```python
from build123d import *

# Parameters (mm, degrees)
F1_DEPTH = 20
F2_DEPTH = 5
F3_W     = 60
F3_H     = 100
F4_DEPTH = 0.5


with BuildPart() as f1:
    # F0 (on Top) → F1 (new body)
    with BuildSketch(Plane.XY):
        with BuildLine():
            Line((45, -47.5), (45, 47.5))
            ThreePointArc((45, 47.5), (39.874369, 59.874369), (27.5, 65))
            Line((27.5, 65), (-27.5, 65))
            ThreePointArc((-27.5, 65), (-39.874369, 59.874369), (-45, 47.5))
            Line((-45, 47.5), (-45, -47.5))
            ThreePointArc((-45, -47.5), (-39.874369, -59.874369), (-27.5, -65))
            Line((-27.5, -65), (27.5, -65))
            ThreePointArc((27.5, -65), (39.874369, -59.874369), (45, -47.5))
        make_face()
        with BuildLine():
            Line((-27.5, 62.5), (27.5, 62.5))
            ThreePointArc((27.5, 62.5), (38.106602, 58.106602), (42.5, 47.5))
            Line((42.5, 47.5), (42.5, -47.5))
            ThreePointArc((42.5, -47.5), (38.106602, -58.106602), (27.5, -62.5))
            Line((27.5, -62.5), (-27.5, -62.5))
            ThreePointArc((-27.5, -62.5), (-38.106602, -58.106602), (-42.5, -47.5))
            Line((-42.5, -47.5), (-42.5, 47.5))
            ThreePointArc((-42.5, 47.5), (-38.106602, 58.106602), (-27.5, 62.5))
        make_face(mode=Mode.SUBTRACT)
    extrude(amount=F1_DEPTH)

    # F0 (on Top) → F2 (join)
    with BuildSketch(Plane.XY):
        with BuildLine():
            ThreePointArc((42.5, 47.5), (38.106602, 58.106602), (27.5, 62.5))
            Line((27.5, 62.5), (-27.5, 62.5))
            ThreePointArc((-27.5, 62.5), (-38.106602, 58.106602), (-42.5, 47.5))
            Line((-42.5, 47.5), (-42.5, -47.5))
            ThreePointArc((-42.5, -47.5), (-38.106602, -58.106602), (-27.5, -62.5))
            Line((-27.5, -62.5), (27.5, -62.5))
            ThreePointArc((27.5, -62.5), (38.106602, -58.106602), (42.5, -47.5))
            Line((42.5, -47.5), (42.5, 47.5))
        make_face()
        with BuildLine():
            Line((-20, 47.5), (20, 47.5))
            ThreePointArc((20, 47.5), (25.303301, 45.303301), (27.5, 40))
            Line((27.5, 40), (27.5, -40))
            ThreePointArc((27.5, -40), (25.303301, -45.303301), (20, -47.5))
            Line((20, -47.5), (-20, -47.5))
            ThreePointArc((-20, -47.5), (-25.303301, -45.303301), (-27.5, -40))
            Line((-27.5, -40), (-27.5, 40))
            ThreePointArc((-27.5, 40), (-25.303301, 45.303301), (-20, 47.5))
        make_face(mode=Mode.SUBTRACT)
        with BuildLine():
            ThreePointArc((27.5, 40), (25.303301, 45.303301), (20, 47.5))
            Line((20, 47.5), (-20, 47.5))
            ThreePointArc((-20, 47.5), (-25.303301, 45.303301), (-27.5, 40))
            Line((-27.5, 40), (-27.5, -40))
            ThreePointArc((-27.5, -40), (-25.303301, -45.303301), (-20, -47.5))
            Line((-20, -47.5), (20, -47.5))
            ThreePointArc((20, -47.5), (25.303301, -45.303301), (27.5, -40))
            Line((27.5, -40), (27.5, 40))
        make_face()
        with BuildLine():
            ThreePointArc((20, 45), (23.535534, 43.535534), (25, 40))
            Line((25, 40), (25, -40))
            ThreePointArc((25, -40), (23.535534, -43.535534), (20, -45))
            Line((20, -45), (-20, -45))
            ThreePointArc((-20, -45), (-23.535534, -43.535534), (-25, -40))
            Line((-25, -40), (-25, 40))
            ThreePointArc((-25, 40), (-23.535534, 43.535534), (-20, 45))
            Line((-20, 45), (20, 45))
        make_face(mode=Mode.SUBTRACT)
    extrude(amount=F2_DEPTH)

    # F3 (on face) → F4 (join)
    with BuildSketch(Plane.XY.offset(5)):
        Rectangle(F3_W, F3_H)
    extrude(amount=F4_DEPTH)


solid = f1.part
```
Geometry: final body of the model. Coordinates: model frame, mm. A direction names the side the tool comes from. Give positions to 0.01 mm unless a question says otherwise; leave off trailing zeros. Write each loop counter-clockwise with the first axis right and the second up, starting at its lowest first coordinate (ties: lowest second). Pieces come first, ordered by that corner, then holes.
1. Line query: probe 1 along Y at (x, z) = (14, 6); probe 2 along X at (y, z) = (15, 1); probe 3 along X at (y, z) = (39, 12.5). Output: solid intervals per line, ascending.
2. Section query A-A, the plane y = 27. Return loops of the section in (x, z), then the cut area to 3 significant figures.
3. Section query D-D, the plane y = -53. Return loops of the section in (x, z), then the cut area to 3 significant figures.
4. Reachability of faces 4 (the flat face through (0, 1, 5)), 5 (the flat face through (43, 15, 20)), 6 (the flat face through (-42.5, -1, 12)) from +Z, -Z, +X, -X, +Y, -Y: full face, straight path, thin tool, end or side. Return the list, or none.
5. Draft query along Y for faces 1 (the flat face through (0, -65, 10)), 2 (the flat face through (0, 65, 10)), 3 (the cylindrical face through (-24, 43, 2)). Return one class per face: released by +Y, released by -Y, zero draft, split by the parting line, or undercut.
6. Pin query (flat end, axial travel): P1, Ø18, axis at x = 1.5, y = -22, coming from the +Z side. Return the tip coordinate at first contact, or that it passes through.
7. Section query B-B, the plane z = 1.75. Return loops of the section in (x, y), then the cut area to 3 significant figures.
8. Section query C-C, the plane x = -9. Return loops of the section in (y, z).
Computed:
1. probe 1: y = -65 to -62.5, 62.5 to 65
1. probe 2: x = -45 to -25, 25 to 45
1. probe 3: x = -45 to -42.5, 42.5 to 45
2. outline: (-45, 0) - (-25, 0) - (-25, 5) - (25, 5) - (25, 0) - (45, 0) - (45, 20) - (42.5, 20) - (42.5, 5) - (30, 5) - (30, 5.5) - (-30, 5.5) - (-30, 5) - (-42.5, 5) - (-42.5, 20) - (-45, 20) - close
2. area: 305 mm2
3. outline: (-44.11, 0) - (44.11, 0) - (44.11, 20) - (41.46, 20) - (41.46, 5) - (-41.46, 5) - (-41.46, 20) - (-44.11, 20) - close
3. area: 521 mm2
4. face 4: -Z
4. face 5: +Z, +X, -X, +Y, -Y
4. face 6: +Z
5. face 1: released by -Y
5. face 2: released by +Y
5. face 3: undercut
6. P1: stops at z = 5.5
7. outline: (-45, -47.5) arc R17.5 ccw to (-27.5, -65) - (27.5, -65) arc R17.5 ccw to (45, -47.5) - (45, 47.5) arc R17.5 ccw to (27.5, 65) - (-27.5, 65) arc R17.5 ccw to (-45, 47.5) - close; hole (-25, -40) arc R5 ccw to (-20, -45) - (20, -45) arc R5 ccw to (25, -40) - (25, 40) arc R5 ccw to (20, 45) - (-20, 45) arc R5 ccw to (-25, 40) - close
7. area: 6,960 mm2
8. outline: (-65, 0) - (-45, 0) - (-45, 5) - (45, 5) - (45, 0) - (65, 0) - (65, 20) - (62.5, 20) - (62.5, 5) - (50, 5) - (50, 5.5) - (-50, 5.5) - (-50, 5) - (-62.5, 5) - (-62.5, 20) - (-65, 20) - close
